Part model, mm, in its own coordinate system. Give positions to 0.01 mm unless a question says otherwise; leave off trailing zeros. Write each loop counter-clockwise with the first axis right and the second up, starting at its lowest first coordinate (ties: lowest second). Pieces come first, ordered by that corner, then holes. Notation, with made-up numbers: M 27,-20.75 L 82,-20.75 A13 cw 82,-5.75 Z; hole C 36,50.25 d1. An arc over 180 degrees is marked long. Write item = value, one per line. Start each with the question number.
from build123d import *

# Parameters (mm, degrees)
F1_DEPTH = 25.4


with BuildPart() as f1:
    # F0 (on Front) → F1 (new body)
    with BuildSketch(Plane.XZ):
        with BuildLine():
            ThreePointArc((-1108.766913414, 0), (-836.979746873, -130.3325864651), (-579.9417495728, -287.7692878246))
            ThreePointArc((-579.9417495728, -287.7692878246), (-186.6180808752, -352.1716385989), (0, 0))
            ThreePointArc((0, 0), (-554.383456707, -29.0433212184), (-1108.766913414, 0))
        make_face()
        with BuildLine():
            Line((-834.7774703357, -268.5709603033), (-579.9417495728, -287.7692878246))
            ThreePointArc((-579.9417495728, -287.7692878246), (-836.979746873, -130.3325864651), (-1108.766913414, 0))
            ThreePointArc((-1108.766913414, 0), (-1000.6160082702, -163.7112273788), (-834.7774703357, -268.5709603032))
        make_face()
        with BuildLine():
            ThreePointArc((-834.7774703357, -268.5709603032), (-708.6979426518, -295.9349516107), (-579.9417495728, -287.7692878246))
            Line((-579.9417495728, -287.7692878246), (-834.7774703357, -268.5709603033))
        make_face()
        with BuildLine():
            ThreePointArc((-834.7774703357, -268.5709603032), (-1000.6160082702, -163.7112273788), (-1108.766913414, 0))
            ThreePointArc((-1108.766913414, 0), (-1186.9150728411, -168.7262748124), (-1362.894263815, -228.784704513))
            Line((-1362.894263815, -228.784704513), (-834.7774703357, -268.5709603033))
        make_face()
        with BuildLine():
            ThreePointArc((-1362.894263815, -228.784704513), (-1186.9150728411, -168.7262748124), (-1108.766913414, 0))
            Line((-1108.766913414, 0), (-1581.4932584763, 0))
            Line((-1581.4932584763, 0), (-1362.894263815, -228.784704513))
        make_face()
        with BuildLine():
            Line((-2085.1438045502, -228.784704513), (-1362.894263815, -228.784704513))
            ThreePointArc((-1362.894263815, -228.784704513), (-1416.5381040648, -218.4133648746), (-1466.3696860565, -196.0071220202))
            Line((-1466.3696860565, -196.0071220202), (-2085.1438045502, 0))
            Line((-2085.1438045502, 0), (-2085.1438045502, -228.784704513))
        make_face()
        with BuildLine():
            Line((-1466.3696860565, -196.0071220202), (-1362.894263815, -228.784704513))
            Line((-1362.894263815, -228.784704513), (-1581.4932584763, 0))
            ThreePointArc((-1581.4932584763, 0), (-1549.0286727991, -112.7442467223), (-1466.3696860565, -196.0071220202))
        make_face()
        with BuildLine():
            ThreePointArc((-1466.3696860565, -196.0071220202), (-1416.5381040648, -218.4133648746), (-1362.894263815, -228.784704513))
            Line((-1362.894263815, -228.784704513), (-1466.3696860565, -196.0071220202))
        make_face()
        with BuildLine():
            ThreePointArc((-1466.3696860565, -196.0071220202), (-1549.0286727991, -112.7442467223), (-1581.4932584763, 0))
            Line((-1581.4932584763, 0), (-2085.1438045502, 0))
            Line((-2085.1438045502, 0), (-1466.3696860565, -196.0071220202))
        make_face()
        with BuildLine():
            Line((-2074.405670166, -246.9456195831), (-2085.1438045502, -228.784704513))
            Line((-2085.1438045502, -228.784704513), (-2085.1438045502, 0))
            ThreePointArc((-2085.1438045502, 0), (-2346.5898933402, -135.0749471589), (-2074.405670166, -246.9456195831))
        make_face()
    extrude(amount=F1_DEPTH)


solid = f1.part
Q1. Slice it at A-A (y = -15.25). Give the cut face in (x, z).
Q2. Drop flat-ended pins along their axis: P1, Ø1.5, axis at y = -22.5, z = -321.5, coming from the +X side; P2, Ø12, axis at x = -1074.5, z = -260.5, coming from the +Y side; P3, Ø6, axis at x = -1812, y = -9.5, coming from the -Z side; P4, Ø8, axis at y = -8, z = -261.5, coming from the -X side. Give the stop position or say it passes through.
Q3. Two-plate mould, pull along X, no slides. Class faces 1 (the face through (-1102.5, -12.5, -248.4)), 2 (the face through (-1188, 0, -127)): +X half, -X half, draft (parallel to the pull), parting line (faces both ways), or undercut.
Q4. Slice it at C-C (z = -316.5). Give the cut face in (x, y).
Q5. Slice it at B-B (x = -1388). Give the cut face in (y, z).
Q6. Probe line 1 along Z through (x, y) = (-1652, -10.5); line 2 along Z through (x, y) = (-359.5, -10); line 3 along X through (y, z) = (-9, -300). List the from-to ranges inside material, lowest first.
Working result:
q1.outline = M -2085.14,-228.78 L -1362.89,-228.78 L -834.78,-268.57 A467.15 ccw -579.94,-287.77 A341.59 ccw 0,0 A5305.6 cw -1108.77,0 L -2085.14,0 A162.13 ccw long -2074.41,-246.95 Z
q2.P1 = -135.24
q2.P2 = through
q2.P3 = -228.78
q2.P4 = -2282.2
q3.face_1 = undercut
q3.face_2 = draft
q4.outline = M -547.28,-25.4 L -129.62,-25.4 L -129.62,0 L -547.28,0 Z
q5.outline = M -25.4,-228.78 L 0,-228.78 L 0,0 L -25.4,0 Z
q6.line_1 = -228.78 to 0
q6.line_2 = -387.12 to -25.46
q6.line_3 = -567.05 to -109.85
